Check sheet for the modelled part. Datum: model origin and axes. Units: mm. Face numbers are marked on the shaded views. A direction names the side the tool comes from. Give positions to 0.01 mm unless a question says otherwise; leave off trailing zeros. Write each loop counter-clockwise with the first axis right and the second up, starting at its lowest first coordinate (ties: lowest second). Pieces come first, ordered by that corner, then holes.
from build123d import *

# Parameters (mm, degrees)
F0_W          = 211.83
F0_H          = 132
F1_DEPTH      = 310
F1_DEPTH_BACK = 160
F2_W          = 32.95
F2_H          = 132
F2_R          = 6
F2_R_2        = 5
F3_DEPTH      = 5
F4_SIZE       = 5
F5_W          = 310
F5_H          = 353
F6_DEPTH      = 50
F7_SIZE       = 15
F8_W          = 310
F8_H          = 110
F8_R          = 11
F8_R_2        = 6
F9_DEPTH      = 10
F10_SIZE      = 8


with BuildPart() as f1:
    # F0 (on Right) → F1 (new body, two sides)
    with BuildSketch(Plane.YZ) as f1_sk:
        with Locations((0, -29.678499)):
            Rectangle(F0_W, F0_H)
    extrude(amount=F1_DEPTH)
    extrude(f1_sk.sketch, amount=-F1_DEPTH_BACK)

    # F2 (on face) → F3 (join)
    with BuildSketch(Plane(origin=(-160, 0, 0), x_dir=(0, -1, 0), z_dir=(-1, 0, 0))):
        with Locations((-89.44, -29.678499)):
            Rectangle(F2_W, F2_H)
        with Locations((-89.44, -79.678499)):
            Circle(F2_R, mode=Mode.SUBTRACT)
        with Locations((-89.44, -29.678499)):
            Circle(F2_R_2, mode=Mode.SUBTRACT)
        with Locations((-89.44, 20.321501)):
            Circle(F2_R, mode=Mode.SUBTRACT)
        with Locations((89.44, -29.678499)):
            Rectangle(F2_W, F2_H)
        with Locations((89.44, -79.678499)):
            Circle(F2_R, mode=Mode.SUBTRACT)
        with Locations((89.44, -29.678499)):
            Circle(F2_R_2, mode=Mode.SUBTRACT)
        with Locations((89.44, 20.321501)):
            Circle(F2_R, mode=Mode.SUBTRACT)
    extrude(amount=F3_DEPTH)

    # F4
    f4_edges = [f1.edges().sort_by_distance(p)[0] for p in [
        (310, 0, 36.321501),
        (72.5, -105.915, 36.321501),
        (72.5, 105.915, 36.321501),
    ]]
    chamfer(f4_edges, length=F4_SIZE)

    # F5 (on face) → F6 (join)
    with BuildSketch(Plane(origin=(0, 0, -95.678499), x_dir=(1, 0, 0), z_dir=(0, 0, -1))):
        with Locations((155, 0)):
            Rectangle(F5_W, F5_H)
    extrude(amount=F6_DEPTH)

    # F7
    f7_edges = [f1.edges().sort_by_distance(p)[0] for p in [
        (155, -176.5, -95.678499),
        (155, 176.5, -95.678499),
    ]]
    chamfer(f7_edges, length=F7_SIZE)

    # F8 (on face) → F9 (join)
    with BuildSketch(Plane(origin=(0, 0, -145.678499), x_dir=(1, 0, 0), z_dir=(0, 0, -1))):
        with Locations((155, 121.5)):
            Rectangle(F8_W, F8_H)
        with Locations((40.08206, 121.5)):
            Circle(F8_R, mode=Mode.SUBTRACT)
        with Locations((155, 121.5)):
            Circle(F8_R_2, mode=Mode.SUBTRACT)
        with Locations((269.91794, 121.5)):
            Circle(F8_R, mode=Mode.SUBTRACT)
        with Locations((155, -121.5)):
            Rectangle(F8_W, F8_H)
        with Locations((40.08206, -121.5)):
            Circle(F8_R, mode=Mode.SUBTRACT)
        with Locations((155, -121.5)):
            Circle(F8_R_2, mode=Mode.SUBTRACT)
        with Locations((269.91794, -121.5)):
            Circle(F8_R, mode=Mode.SUBTRACT)
    extrude(amount=F9_DEPTH)

    # F10
    f10_edges = [f1.edges().sort_by_distance(p)[0] for p in [
        (0, -176.5, -133.178499),
        (0, 176.5, -133.178499),
        (310, 176.5, -133.178499),
        (310, -176.5, -133.178499),
    ]]
    chamfer(f10_edges, length=F10_SIZE)


solid = f1.part
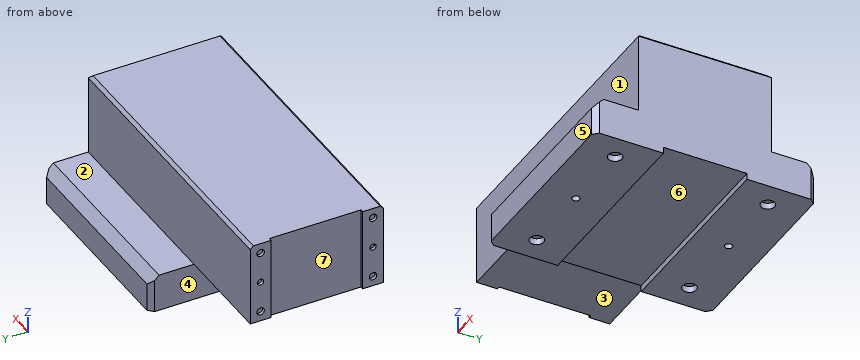
1) Sectioned sample at C-C on z = -133. Record the boundary of the cut face in (x, y), then the cut area to 3 significant figures.
2) Draft check along Y on the marked faces 4, 5, 6 and 7. Enter one of: +Y half, -Y half, draft (parallel to the pull), parting line (faces both ways), or undercut.
3) Gauge pin test, flat ends, axial feed: pin 1 (8 mm diameter, centred on y = 63.5, z = -101.5, fed in from -X); pin 2 (20 mm diameter, centred on x = 40.08, y = -121.5, fed in from -Z); pin 3 (7 mm diameter, centred on y = -89.44, z = 20.32, fed in from -X). Record the tip position at first contact, or that the pin passes through.
4) Scan lines: L1, parallel to Z at x = -163, y = -89; L2, parallel to X at y = -121, z = -149; L3, parallel to Z at x = 290, y = 101. Record each from-to range of solid material in increasing order.
5) Sectioned sample at D-D on y = 0.5. Record the boundary of the cut face in (x, z), then the cut area to 3 significant figures.
6) Sectioned sample at B-B on y = 89.44. Record the boundary of the cut face in (x, z).
7) Sectioned sample at A-A on x = 172.5. Record the boundary of the cut face in (y, z) (1 decimal), then the cut area to 3 significant figures.
8) Access from +Z, -Z, +X, -X, +Y, -Y to the whole of each face (thin tool, end or side, straight path). Record for the marked faces 1, 2 and 3.
Answers below:
1. outline: (0, -168.5) - (8, -176.5) - (302, -176.5) - (310, -168.5) - (310, 168.5) - (302, 176.5) - (8, 176.5) - (0, 168.5) - close
1. area: 109,000 mm2
2. face 4: draft
2. face 5: -Y half
2. face 6: undercut
2. face 7: undercut
3. pin 1: stops at x = 0
3. pin 2: stops at z = -145.68
3. pin 3: stops at x = -160
4. L1: z = -95.68 to -85.66, -73.69 to -34.66, -24.7 to 14.34, 26.31 to 36.32
4. L2: x = 0 to 29.09, 51.07 to 149.02, 160.98 to 258.93, 280.91 to 310
4. L3: z = -155.68 to 36.24
5. outline: (-160, -95.68) - (0, -95.68) - (0, -145.68) - (310, -145.68) - (310, 31.32) - (305, 36.32) - (-160, 36.32) - close
5. area: 77,500 mm2
6. outline: (-165, -95.68) - (0, -95.68) - (0, -155.68) - (310, -155.68) - (310, 31.32) - (305, 36.32) - (-165, 36.32) - (-165, 26.32) - (-160, 26.32) - (-160, 14.32) - (-165, 14.32) - (-165, -24.68) - (-160, -24.68) - (-160, -34.68) - (-165, -34.68) - (-165, -73.68) - (-160, -73.68) - (-160, -85.68) - (-165, -85.68) - close
7. outline: (-176.5, -155.7) - (-66.5, -155.7) - (-66.5, -145.7) - (66.5, -145.7) - (66.5, -155.7) - (176.5, -155.7) - (176.5, -110.7) - (161.5, -95.7) - (105.9, -95.7) - (105.9, 31.3) - (100.9, 36.3) - (-100.9, 36.3) - (-105.9, 31.3) - (-105.9, -95.7) - (-161.5, -95.7) - (-176.5, -110.7) - close
7. area: 47,600 mm2
8. face 1: +Z, +X, -X, -Y
8. face 2: +Z, +X, -X, +Y
8. face 3: -Z, -X, +Y, -Y
